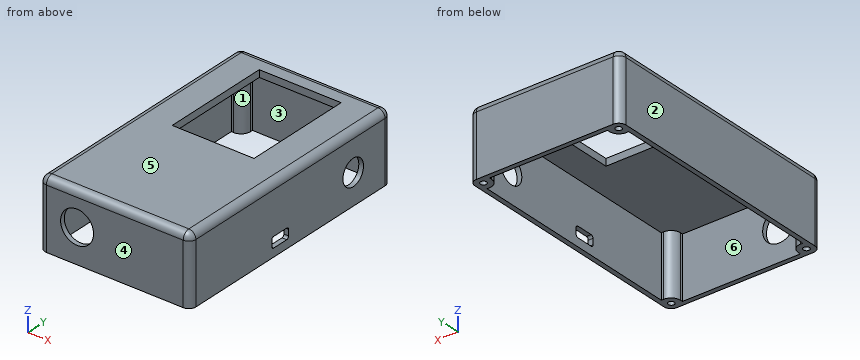
from build123d import *

# Parameters (mm, degrees)
ESQUISSE1_W             = 60
ESQUISSE1_H             = 103
BOSS_EXTRU_1_DEPTH      = 3
ESQUISSE2_W             = 34.7
ESQUISSE2_H             = 46.5
ENL_V_MAT_EXTRU_1_DEPTH = 120.239255281
ESQUISSE3_W             = 41
ESQUISSE3_H             = 2.8
ENL_V_MAT_EXTRU_2_DEPTH = 1.8
BOSS_EXTRU_2_DEPTH      = 26
BOSS_EXTRU_2_DEPTH_BACK = 3
ESQUISSE4_W             = 64
ESQUISSE4_H             = 107
ESQUISSE4_W_2           = 60
ESQUISSE4_H_2           = 103
ENL_V_MAT_EXTRU_3_REACH = 127.686
ESQUISSE5_R             = 5.5
ESQUISSE5_W             = 4.5
ESQUISSE5_H             = 9
CONG_1_R                = 1
CONG_2_R                = 3
ESQUISSE6_W             = 5
ESQUISSE6_H             = 5
BOSS_EXTRU_3_DEPTH      = 26
CONG_3_R                = 4
ESQUISSE7_R             = 1.3
ENL_V_MAT_EXTRU_4_DEPTH = 10
ENL_V_MAT_EXTRU_5_REACH = 128.369
ESQUISSE8_R             = 7


with BuildPart() as part:
    # Esquisse1 → Boss.-Extru.1 (new body)
    with BuildSketch(Plane.XY):
        with Locations((30, 51.5)):
            Rectangle(ESQUISSE1_W, ESQUISSE1_H)
    extrude(amount=BOSS_EXTRU_1_DEPTH)

    # Esquisse2 → Enlèv. mat.-Extru.1 (cut, through all)
    with BuildSketch(Plane.XY.offset(3)):
        with Locations((30, 73.75)):
            Rectangle(ESQUISSE2_W, ESQUISSE2_H)
    extrude(amount=-ENL_V_MAT_EXTRU_1_DEPTH, mode=Mode.SUBTRACT)

    # Esquisse3 → Enlèv. mat.-Extru.2 (cut)
    with BuildSketch(Plane(origin=(0, 0, 0), x_dir=(-1, 0, 0), z_dir=(0, 0, -1))):
        with Locations((-30, 99.6)):
            Rectangle(ESQUISSE3_W, ESQUISSE3_H)
    extrude(amount=-ENL_V_MAT_EXTRU_2_DEPTH, mode=Mode.SUBTRACT)

    # Esquisse4 → Boss.-Extru.2 (add, two sides: drawn at the far end of the back side and taken through both)
    with BuildSketch(Plane(origin=(0, 0, 0), x_dir=(-1, 0, 0), z_dir=(0, 0, -1)).offset(-BOSS_EXTRU_2_DEPTH_BACK)):
        with Locations((-30, 51.5)):
            Rectangle(ESQUISSE4_W, ESQUISSE4_H)
        with Locations((-30, 51.5)):
            Rectangle(ESQUISSE4_W_2, ESQUISSE4_H_2, mode=Mode.SUBTRACT)
    extrude(amount=BOSS_EXTRU_2_DEPTH + BOSS_EXTRU_2_DEPTH_BACK)

    # Esquisse5 → Enlèv. mat.-Extru.3 (cut, up to next)
    with BuildSketch(Plane(origin=(62, 0, 0), x_dir=(0, 0, -1), z_dir=(1, 0, 0)), mode=Mode.PRIVATE) as enl_v_mat_extru_3_sk1:
        with Locations(Location((13, 85, 0), (0, 0, 90))):
            Circle(ESQUISSE5_R)
    enl_v_mat_extru_3_tool1 = extrude(enl_v_mat_extru_3_sk1.sketch, amount=-ENL_V_MAT_EXTRU_3_REACH, mode=Mode.PRIVATE) & part.part
    # Esquisse5 → Enlèv. mat.-Extru.3 (cut, up to next)
    with BuildSketch(Plane(origin=(62, 0, 0), x_dir=(0, 0, -1), z_dir=(1, 0, 0)), mode=Mode.PRIVATE) as enl_v_mat_extru_3_sk2:
        with Locations((20.25, 46)):
            Rectangle(ESQUISSE5_W, ESQUISSE5_H)
    enl_v_mat_extru_3_tool2 = extrude(enl_v_mat_extru_3_sk2.sketch, amount=-ENL_V_MAT_EXTRU_3_REACH, mode=Mode.PRIVATE) & part.part
    add(enl_v_mat_extru_3_tool1.solids().sort_by_distance((62, 85, -13))[0], mode=Mode.SUBTRACT)
    add(enl_v_mat_extru_3_tool2.solids().sort_by_distance((62, 46, -20.25))[0], mode=Mode.SUBTRACT)

    # Congé1
    cong_1_edges = [part.edges().sort_by_distance(p)[0] for p in [
        (61, 41.5, -18),
        (61, 50.5, -18),
        (61, 50.5, -22.5),
        (61, 41.5, -22.5),
    ]]
    fillet(cong_1_edges, radius=CONG_1_R)

    # Congé2
    cong_2_edges = [part.edges().sort_by_distance(p)[0] for p in [
        (-2, 105, -11.5),
        (-2, 51.5, 3),
        (-2, -2, -11.5),
        (30, -2, 3),
        (62, -2, -11.5),
        (62, 51.5, 3),
        (62, 105, -11.5),
        (30, 105, 3),
    ]]
    fillet(cong_2_edges, radius=CONG_2_R)

    # Esquisse6 → Boss.-Extru.3 (add)
    with BuildSketch(Plane(origin=(0, 0, -26), x_dir=(-1, 0, 0), z_dir=(0, 0, -1))):
        with Locations((-57.5, 100.5)):
            Rectangle(ESQUISSE6_W, ESQUISSE6_H)
        with Locations((-2.5, 100.5)):
            Rectangle(ESQUISSE6_W, ESQUISSE6_H)
        with Locations((-2.5, 2.5)):
            Rectangle(ESQUISSE6_W, ESQUISSE6_H)
        with Locations((-57.5, 2.5)):
            Rectangle(ESQUISSE6_W, ESQUISSE6_H)
    extrude(amount=-BOSS_EXTRU_3_DEPTH)

    # Congé3
    cong_3_edges = [part.edges().sort_by_distance(p)[0] for p in [
        (55, 98, -13),
        (5, 98, -13),
        (5, 5, -13),
        (55, 5, -13),
    ]]
    fillet(cong_3_edges, radius=CONG_3_R)

    # Esquisse7 → Enlèv. mat.-Extru.4 (cut)
    with BuildSketch(Plane(origin=(0, 0, -26), x_dir=(-1, 0, 0), z_dir=(0, 0, -1))):
        with Locations((-1.353553391, 101.646446609)):
            Circle(ESQUISSE7_R)
        with Locations(Location((-58.646446609, 101.646446609, 0), (0, 0, 180))):
            Circle(ESQUISSE7_R)
        with Locations((-58.646446609, 1.353553391)):
            Circle(ESQUISSE7_R)
        with Locations(Location((-1.353553391, 1.353553391, 0), (0, 0, 180))):
            Circle(ESQUISSE7_R)
    extrude(amount=-ENL_V_MAT_EXTRU_4_DEPTH, mode=Mode.SUBTRACT)

    # Esquisse8 → Enlèv. mat.-Extru.5 (cut, up to next)
    with BuildSketch(Plane(origin=(0, -2, 0), x_dir=(-1, 0, 0), z_dir=(0, -1, 0)), mode=Mode.PRIVATE) as enl_v_mat_extru_5_sk1:
        with Locations(Location((-14, 11.5, 0), (0, 0, 180))):
            Circle(ESQUISSE8_R)
    enl_v_mat_extru_5_tool1 = extrude(enl_v_mat_extru_5_sk1.sketch, amount=-ENL_V_MAT_EXTRU_5_REACH, mode=Mode.PRIVATE) & part.part
    add(enl_v_mat_extru_5_tool1.solids().sort_by_distance((14, -2, -11.5))[0], mode=Mode.SUBTRACT)


solid = part.part
Geometry: final body of the model. Coordinates: model frame, mm. Face numbers are marked on the shaded views. A direction names the side the tool comes from. Coordinates: 2 decimals unless noted, no trailing zeros. Write each loop counter-clockwise with the first axis right and the second up, starting at its lowest first coordinate (ties: lowest second). Pieces come first, ordered by that corner, then holes. Notation, with made-up numbers: (12, 57.25) - (62, 57.25) arc R15 ccw to (62, 62.25) - close; hole circle Ø4 at (39, 53.5). An arc over 180 degrees is marked (long way). Return JSON: item names as keys, results as strings.
Item 1: Line query: L1, parallel to X at y = 26, z = -13.75; L2, parallel to Y at x = 8.5, z = -17; L3, parallel to Y at x = 39, z = 1. Output: solid intervals per line, ascending.
Completed:
{"L1": "x = -2 to 0, 60 to 62", "L2": "y = -2 to 0, 103 to 105", "L3": "y = -1.83 to 50.5, 97 to 98.2, 101 to 104.83"}
Item 2: Pin query (flat end, axial travel): pin 1 Ø1.4 at (y, z) = (100, 1) entering from +X; pin 2 Ø2.5 at (y, z) = (79, 1.5) entering from -X; pin 3 Ø2 at (x, y) = (61, 46.5) entering from +Z. Return the tip coordinate at first contact, or that it passes through.
Completed:
{"pin 1": "stops at x = 61.98", "pin 2": "stops at x = -1.99", "pin 3": "stops at z = 2.83"}
Item 3: Section query D-D (y = 57). Output: boundary loops of the cut face in (x, z).
Completed:
{"outline": "(-2, -26) - (0, -26) - (0, 0) - (12.65, 0) - (12.65, 3) - (1, 3) arc R3 ccw to (-2, 0) - close; (47.35, 0) - (60, 0) - (60, -26) - (62, -26) - (62, 0) arc R3 ccw to (59, 3) - (47.35, 3) - close"}
Item 4: Section query B-B (y = 85). Output: boundary loops of the cut face in (x, z).
Completed:
{"outline": "(-2, -26) - (0, -26) - (0, 0) - (12.65, 0) - (12.65, 3) - (1, 3) arc R3 ccw to (-2, 0) - close; (47.35, 0) - (60, 0) - (60, -7.5) - (62, -7.5) - (62, 0) arc R3 ccw to (59, 3) - (47.35, 3) - close; (60, -26) - (62, -26) - (62, -18.5) - (60, -18.5) - close"}
Item 5: Pull-direction query (Y, two-part tool) for the marked faces 3, 4, 5 and 6; classes: +Y half, -Y half, draft (parallel to the pull), parting line (faces both ways), or undercut.
Completed:
{"face 3": "undercut", "face 4": "-Y half", "face 5": "draft", "face 6": "undercut"}
Item 6: Reachability of the marked faces 1 and 2 from +Z, -Z, +X, -X, +Y, -Y: full face, straight path, thin tool, end or side. Return the list, or none.
Completed:
{"face 1": "-Z", "face 2": "+Z, -Z, -X, +Y, -Y"}
Item 7: Section query A-A (x = 37). Output: boundary loops of the cut face in (y, z).
Completed:
{"outline": "(-2, -26) - (0, -26) - (0, 0) - (50.5, 0) - (50.5, 3) - (1, 3) arc R3 ccw to (-2, 0) - close; (97, 0) - (98.2, 0) - (98.2, 1.8) - (101, 1.8) - (101, 0) - (103, 0) - (103, -26) - (105, -26) - (105, 0) arc R3 ccw to (102, 3) - (97, 3) - close"}
Item 8: Section query C-C (x = 14). Output: boundary loops of the cut face in (y, z).
Completed:
{"outline": "(-2, -26) - (0, -26) - (0, -18.5) - (-2, -18.5) - close; (-2, -4.5) - (0, -4.5) - (0, 0) - (50.5, 0) - (50.5, 3) - (1, 3) arc R3 ccw to (-2, 0) - close; (97, 0) - (98.2, 0) - (98.2, 1.8) - (101, 1.8) - (101, 0) - (103, 0) - (103, -26) - (105, -26) - (105, 0) arc R3 ccw to (102, 3) - (97, 3) - close"}
